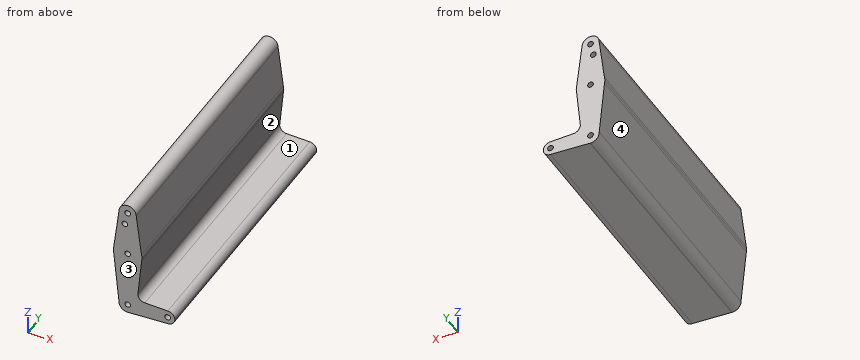
from build123d import *

# Parameters (mm, degrees)
F0_R     = 3.175
F1_DEPTH = 304.8


with BuildPart() as f1:
    # F0 (on Front) → F1 (new body)
    with BuildSketch(Plane.XZ):
        with BuildLine():
            ThreePointArc((-9.525, 114.3), (0, 104.775), (9.525, 114.3))
            ThreePointArc((9.525, 114.3), (0, 123.825), (-9.525, 114.3))
        make_face()
        with Locations((0, 114.3)):
            Circle(F0_R, mode=Mode.SUBTRACT)
        with BuildLine():
            Line((15.3865384615, 67.4076923077), (9.525, 114.3))
            ThreePointArc((9.525, 114.3), (0, 104.775), (-9.525, 114.3))
            Line((-9.525, 114.3), (-15.3865384615, 67.4076923077))
            ThreePointArc((-15.3865384615, 67.4076923077), (0, 79.375), (15.3865384615, 67.4076923077))
        make_face()
        with Locations((-3.175, 99.886942851)):
            Circle(F0_R, mode=Mode.SUBTRACT)
        with BuildLine():
            Line((15.875, 63.5), (15.3865384615, 67.4076923077))
            ThreePointArc((15.3865384615, 67.4076923077), (0, 79.375), (-15.3865384615, 67.4076923077))
            Line((-15.3865384615, 67.4076923077), (-15.875, 63.5))
            Line((-15.875, 63.5), (-15.5652161214, 60.3791552277))
            ThreePointArc((-15.5652161214, 60.3791552277), (0.0227867429, 47.6250163539), (15.5741112031, 60.4238522089))
            Line((15.5741112031, 60.4238522089), (15.875, 63.5))
        make_face()
        with Locations((0, 63.5)):
            Circle(F0_R, mode=Mode.SUBTRACT)
        with BuildLine():
            ThreePointArc((15.875, 63.5), (15.7524112928, 65.4690514116), (15.3865384615, 67.4076923077))
            Line((15.3865384615, 67.4076923077), (15.875, 63.5))
        make_face()
        with BuildLine():
            Line((-15.875, 63.5), (-15.3865384615, 67.4076923077))
            ThreePointArc((-15.3865384615, 67.4076923077), (-15.7524112928, 65.4690514116), (-15.875, 63.5))
        make_face()
        with BuildLine():
            ThreePointArc((15.5741112031, 60.4238522089), (15.7995987346, 61.9545858726), (15.875, 63.5))
            Line((15.875, 63.5), (15.5741112031, 60.4238522089))
        make_face()
        with BuildLine():
            Line((-15.5652161214, 60.3791552277), (-15.875, 63.5))
            ThreePointArc((-15.875, 63.5), (-15.7973641936, 61.9319089516), (-15.5652161214, 60.3791552277))
        make_face()
        with BuildLine():
            Line((11.3902740501, 17.6502376701), (15.5741112031, 60.4238522089))
            ThreePointArc((15.5741112031, 60.4238522089), (0.0227867429, 47.6250163539), (-15.5652161214, 60.3791552277))
            Line((-15.5652161214, 60.3791552277), (-9.6396474759, 0.683408579))
            ThreePointArc((-9.6396474759, 0.683408579), (0.3419183682, 9.6577918064), (9.6638424421, 0))
            ThreePointArc((9.6638424421, 0), (7.0934141051, -6.5630272801), (0.7495151779, -9.6347328839))
            Line((0.7495151779, -9.6347328839), (44.45, -7.9375))
            ThreePointArc((44.45, -7.9375), (36.5127834119, 0.0670752079), (44.584145626, 7.9363663727))
            Line((44.584145626, 7.9363663727), (18.9936011902, 8.9321058415))
            ThreePointArc((18.9936011902, 8.9321058415), (13.311058011, 11.650803927), (11.3902740501, 17.6502376701))
        make_face()
        with BuildLine():
            ThreePointArc((9.6638424421, 0), (0.3419183682, 9.6577918064), (-9.6396474759, 0.683408579))
            ThreePointArc((-9.6396474759, 0.683408579), (-7.0708628744, -6.5873172808), (0, -9.6638424421))
            Line((0, -9.6638424421), (0.7495151779, -9.6347328839))
            ThreePointArc((0.7495151779, -9.6347328839), (7.0934141051, -6.5630272801), (9.6638424421, 0))
        make_face()
        Circle(F0_R, mode=Mode.SUBTRACT)
        with BuildLine():
            Line((0.7495151779, -9.6347328839), (0, -9.6638424421))
            ThreePointArc((0, -9.6638424421), (0.3750401206, -9.6565623104), (0.7495151779, -9.6347328839))
        make_face()
        with BuildLine():
            ThreePointArc((52.3875, 0), (50.1098890076, 5.5650303388), (44.584145626, 7.9363663727))
            ThreePointArc((44.584145626, 7.9363663727), (36.5127834119, 0.0670752079), (44.45, -7.9375))
            ThreePointArc((44.45, -7.9375), (50.0626600757, -5.6126600757), (52.3875, 0))
        make_face()
        with Locations((44.45, 0)):
            Circle(F0_R, mode=Mode.SUBTRACT)
    extrude(amount=F1_DEPTH)


solid = f1.part
Read the model definition and answer for the solid it produces. Units are mm, in the model's axes. Face numbers are marked on the shaded views. Coordinates: 2 decimals unless noted, no trailing zeros. Order: outer loops, then holes, each group sorted by start corner. A loop starts at its lowest first (then second) coordinate and runs counter-clockwise, first axis right, second up. Notation, with made-up numbers: M 39,3.25 L 96,3.25 A20 cw 96,11.25 Z; hole C 50.25,67 d3. An arc over 180 degrees is marked long. Put each result on its own line as item: value. Start each with the question number.
Item 1: Section A-A, the plane y = -233 is taken. Count the separate pieces of the cut face and the enclosed holes in it, plus the area to 3 significant figures.
Item 2: Given pin 1 Ø6 at (x, y) = (21.5, -57.5) entering from +Z; pin 2 Ø7.5 at (x, z) = (0, 0) entering from +Y; pin 3 Ø1 at (y, z) = (-253.5, 33.5) entering from +X; pin 4 Ø3 at (y, z) = (-272, 39) entering from -X, each flat-ended and moving along its own axis, determine where each tip first touches the part or whether it passes through.
Item 3: Consider probe 1 along Z at (x, y) = (2.5, -102.5); probe 2 along X at (y, z) = (-229, 0.5); probe 3 along X at (y, z) = (-135.5, 100). Determine where each line is inside the solid, lowest interval first. Write a range as [from, to].
Item 4: Section B-B, the plane x = 23 is taken. Determine the outline of the cut face in (y, z), plus the area to 3 significant figures.
Item 5: Section C-C, the plane z = 12.5 is taken. Determine the outline of the cut face in (x, y), plus the area to 3 significant figures.
Item 6: The mould has two halves that part along Z. Classify the marked faces 1, 2, 3 and 4: +Z half, -Z half, draft (parallel to the pull), parting line (faces both ways), or undercut.
Computed:
1. separate pieces: 1
1. enclosed holes: 5
1. area: 3,770 mm2
2. pin 1: stops at z = 8.97
2. pin 2: stops at y = 0
2. pin 3: stops at x = 12.99
2. pin 4: stops at x = -13.59
3. probe 1: z = [-9.57, -1.96], [1.96, 61.54], [65.46, 112.34], [116.26, 123.49]
3. probe 2: x = [-9.65, -3.14], [3.14, 41.31], [47.59, 52.37]
3. probe 3: x = [-11.31, -6.35], [0, 11.31]
4. outline: M -304.8,-8.77 L 0,-8.77 L 0,8.78 L -304.8,8.78 Z
4. area: 5,350 mm2
5. outline: M -10.81,-304.8 L 12.67,-304.8 L 12.67,0 L -10.81,0 Z
5. area: 7,160 mm2
6. face 1: +Z half
6. face 2: undercut
6. face 3: draft
6. face 4: -Z half
